The listing builds one solid part. Answer for the finished solid, in the listing's coordinates (mm). Face numbers are marked on the shaded views. Give positions to 0.01 mm unless a question says otherwise; leave off trailing zeros. Loops run counter-clockwise (first coordinate to the right, second up) from the corner with the lowest first, then second, coordinate; pieces in that order, holes last. Notation, with made-up numbers: (41, 76) - (54, 76) arc R16 cw to (54, 92) - close; hole circle Ø11 at (20.5, 36). An arc over 180 degrees is marked (long way). Write item = value, one per line. Start each with the question number.
1) The part is cut by section B-B on z = 0. Write down the section's boundary in (x, y).
2) Flat-ended cylindrical pins translate along their axes: P1, Ø5, axis at x = 0, z = 0, coming from the -Y side; P2, Ø1.5, axis at y = 0, z = 0.5, coming from the -X side; P3, Ø1, axis at y = -0.5, z = 1.5, coming from the -X side. Find the tip coordinate at first contact, or state that the pin passes through.
3) The part is cut by section A-A on x = 0. Write down the section's boundary in (y, z).
4) Consider probe 1 along Y at (x, z) = (-1, -3.25); probe 2 along X at (y, z) = (-1.2, 0); probe 3 along Z at (x, y) = (-3, 0.35). Determine where each line is inside the solid, lowest interval first.
5) The mould has two halves that part along X. Classify the marked faces 1 and 2: +X half, -X half, draft (parallel to the pull), parting line (faces both ways), or undercut.
6) The part is cut by section C-C on y = 2. Write down the section's boundary in (x, z), plus the area to 3 significant figures.
7) The part is cut by section D-D on x = 5. State how many separate pieces and enclosed holes the cut face has, plus the area to 3 significant figures.
from build123d import *

# Parameters (mm, degrees)
SKETCH_3_R      = 1
SKETCH_5_R      = 6
SKETCH_5_R_2    = 3
EXTRUDE_1_DEPTH = 1.5
SKETCH_6_R      = 6
SKETCH_6_R_2    = 5.25
EXTRUDE_3_DEPTH = 1.5
EXTRUDE_START   = 1.5
SKETCH_7_R      = 6
SKETCH_7_R_2    = 3
EXTRUDE_4_DEPTH = 1.5


with BuildPart() as part:
    # Sketch 3 → Revolve 3 (revolve)
    with BuildSketch(Plane(origin=(0, 0, 0), x_dir=(0, 0, -1), z_dir=(1, 0, 0))):
        with Locations((-4.5, 0)):
            Circle(SKETCH_3_R)
    revolve(axis=Axis((0, 7.993421053, 0), (0, -1, 0)))



with BuildPart() as body_2:
    # Sketch 5 → Extrude 1 (new body)
    with BuildSketch(Plane(origin=(0, 0.75, 0), x_dir=(1, 0, 0), z_dir=(0, 1, 0))):
        with Locations(Location((0, 0, 0), (0, 0, 270))):
            Circle(SKETCH_5_R)
        with Locations(Location((0, 0, 0), (0, 0, 270))):
            Circle(SKETCH_5_R_2, mode=Mode.SUBTRACT)
    extrude(amount=EXTRUDE_1_DEPTH)


with BuildPart() as part_1:
    add(part.part)

    add(body_2.part)  # Extrude 3 merges body 2
    # Sketch 6 → Extrude 3 (add)
    with BuildSketch(Plane.XZ.offset(-0.75)):
        with Locations(Location((0, 0, 0), (0, 0, 90))):
            Circle(SKETCH_6_R)
        with Locations(Location((0, 0, 0), (0, 0, 90))):
            Circle(SKETCH_6_R_2, mode=Mode.SUBTRACT)
    extrude(amount=EXTRUDE_3_DEPTH)

    # Sketch 7 → Extrude 4 (add)
    with BuildSketch(Plane.XZ.offset(0.75).offset(EXTRUDE_START)):
        with Locations(Location((0, 0, 0), (0, 0, 90))):
            Circle(SKETCH_7_R)
        with Locations(Location((0, 0, 0), (0, 0, 90))):
            Circle(SKETCH_7_R_2, mode=Mode.SUBTRACT)
    extrude(amount=-EXTRUDE_4_DEPTH)


solid = part_1.part
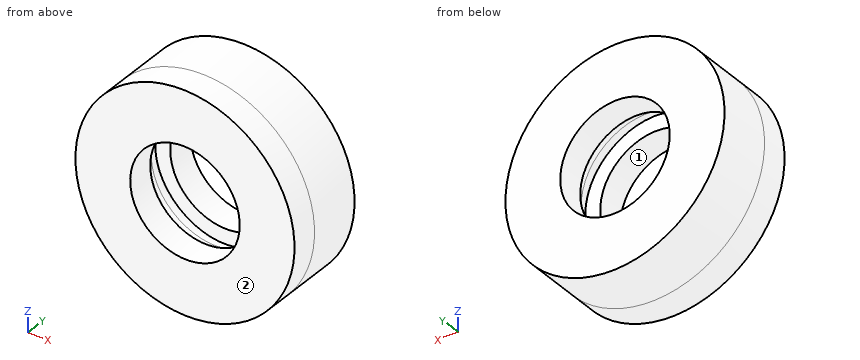
Answer below:
q1.outline = (-6, -2.25) - (-3, -2.25) - (-3, -0.75) - (-3.84, -0.75) arc R1 ccw to (-3.84, 0.75) - (-3, 0.75) - (-3, 2.25) - (-6, 2.25) - close; (3, -2.25) - (6, -2.25) - (6, 2.25) - (3, 2.25) - (3, 0.75) - (3.84, 0.75) arc R1 ccw to (3.84, -0.75) - (3, -0.75) - close; hole (-5.25, -0.75) - (-5.16, -0.75) arc R1 cw to (-5.25, -0.66) - close; hole (-5.25, 0.66) arc R1 cw to (-5.16, 0.75) - (-5.25, 0.75) - close; hole (5.16, -0.75) - (5.25, -0.75) - (5.25, -0.66) arc R1 cw to start; hole (5.16, 0.75) arc R1 cw to (5.25, 0.66) - (5.25, 0.75) - close
q2.P1 = through
q2.P2 = -6
q2.P3 = -5.92
q3.outline = (-2.25, -6) - (2.25, -6) - (2.25, -3) - (0.75, -3) - (0.75, -3.84) arc R1 ccw to (-0.75, -3.84) - (-0.75, -3) - (-2.25, -3) - close; (-2.25, 3) - (-0.75, 3) - (-0.75, 3.84) arc R1 ccw to (0.75, 3.84) - (0.75, 3) - (2.25, 3) - (2.25, 6) - (-2.25, 6) - close; hole (-0.75, -5.25) - (-0.66, -5.25) arc R1 cw to (-0.75, -5.16) - close; hole (-0.75, 5.16) arc R1 cw to (-0.66, 5.25) - (-0.75, 5.25) - close; hole (0.66, -5.25) - (0.75, -5.25) - (0.75, -5.16) arc R1 cw to start; hole (0.66, 5.25) arc R1 cw to (0.75, 5.16) - (0.75, 5.25) - close
q4.probe_1 = -2.25 to -0.75, 0.75 to 2.25
q4.probe_2 = -6 to -3, 3 to 6
q4.probe_3 = -5.2 to -1.92, 1.92 to 5.2
q5.face_1 = undercut
q5.face_2 = draft
q6.outline = circle Ø12 at (0, 0); hole circle Ø6 at (0, 0)
q6.area = 84.8 mm2
q7.separate_pieces = 1
q7.enclosed_holes = 4
q7.area = 29.8 mm2
